The listing builds one solid part. Answer for the finished solid, in the listing's coordinates (mm). A direction names the side the tool comes from. Give positions to 0.01 mm unless a question says otherwise; leave off trailing zeros. Order: outer loops, then holes, each group sorted by start corner. A loop starts at its lowest first (then second) coordinate and runs counter-clockwise, first axis right, second up. Notation, with made-up numbers: (88, -28) -> (92, -28) arc R21 cw to (92, 7) -> close; hole circle Ø6 at (50.25, 0.25). An arc over 180 degrees is marked (long way). Write item = value, one per line. Start each with the question number.
```python
from build123d import *

# Parameters (mm, degrees)
F0_R     = 12.5
F0_R_2   = 11
F1_DEPTH = 5
F0_R_3   = 10.5
F2_DEPTH = 8
F3_DEPTH = 6
F4_D     = 5


with BuildPart() as f1:
    # F0 (on Top) → F1 (new body)
    with BuildSketch(Plane.XY):
        Circle(F0_R)
        Circle(F0_R_2, mode=Mode.SUBTRACT)
    extrude(amount=F1_DEPTH)

    # F0 (on Top) → F2 (join)
    with BuildSketch(Plane.XY):
        Circle(F0_R_2)
        Circle(F0_R_3, mode=Mode.SUBTRACT)
    extrude(amount=F2_DEPTH)

    # F0 (on Top) → F3 (join)
    with BuildSketch(Plane.XY):
        Circle(F0_R_3)
    extrude(amount=F3_DEPTH)

    # F4 (through all)
    with Locations(Plane(origin=(0, 0, 0), x_dir=(1, 0, 0), z_dir=(0, 0, -1))):
        with Locations((0, 0)):
            Hole(F4_D / 2)


solid = f1.part
```
Item 1: A cutting plane is placed at A-A, the plane x = 0. Write down the section's boundary in (y, z), plus the area to 3 significant figures.
Item 2: Which of the six approach directions +Z, -Z, +X, -X, +Y, -Y give full straight-line access (tool end or side, diameter ignored) to faces 4 (the cylindrical face through (0.54, 2.44, 3.04)), 5 (the flat face through (5, -10, 5))?
Item 3: Flat-ended cylindrical pins translate along their axes: pin 1 (6 mm diameter, centred on x = 0.5, y = 7.5, fed in from -Z); pin 2 (1 mm diameter, centred on x = 5.5, z = 3.5, fed in from +Y); pin 3 (8 mm diameter, centred on x = 0, y = 0, fed in from +Z); pin 4 (1 mm diameter, centred on y = 9.5, z = 3, fed in from -X). Find the tip coordinate at first contact, or state that the pin passes through.
Item 4: A cutting plane is placed at C-C, the plane y = 6. Write down the section's boundary in (x, z).
Item 5: The mould has two halves that part along Y. Classify faces 1 (the cylindrical face through (10, 3.2, 7)), 2 (the flat face through (4, -10, 8)), 3 (the cylindrical face through (-2.38, -10.74, 6.48)): +Y half, -Y half, draft (parallel to the pull), parting line (faces both ways), or undercut.
Item 6: Consider L1, parallel to Y at x = 0, z = 7.15; L2, parallel to Y at x = 6.25, z = 7.75; L3, parallel to Z at x = -2.75, y = 2.25. Determine where each line is inside the solid, lowest interval first. Write a range as from..to.
Item 7: A cutting plane is placed at D-D, the plane z = 3.5. Write down the section's boundary in (x, y), plus the area to 3 significant figures.
Check values:
q1.outline = (-12.5, 0) -> (-2.5, 0) -> (-2.5, 6) -> (-10.5, 6) -> (-10.5, 8) -> (-11, 8) -> (-11, 5) -> (-12.5, 5) -> close; (2.5, 0) -> (12.5, 0) -> (12.5, 5) -> (11, 5) -> (11, 8) -> (10.5, 8) -> (10.5, 6) -> (2.5, 6) -> close
q1.area = 119 mm^2
q2.face_4 = +Z, -Z
q2.face_5 = +Z
q3.pin_1 = 0
q3.pin_2 = 11.46
q3.pin_3 = 6
q3.pin_4 = -8.67
q4.outline = (-10.97, 0) -> (10.97, 0) -> (10.97, 5) -> (9.22, 5) -> (9.22, 8) -> (8.62, 8) -> (8.62, 6) -> (-8.62, 6) -> (-8.62, 8) -> (-9.22, 8) -> (-9.22, 5) -> (-10.97, 5) -> close
q5.face_1 = undercut
q5.face_2 = draft
q5.face_3 = parting line
q6.L1 = -11..-10.5, 10.5..11
q6.L2 = -9.05..-8.44, 8.44..9.05
q6.L3 = 0..6
q7.outline = circle Ø25 at (0, 0); hole circle Ø5 at (0, 0)
q7.area = 471 mm^2
